from build123d import *


with BuildPart() as part:
    # Sketch1 → BaseBody (revolve)
    with BuildSketch(Plane.XY, mode=Mode.PRIVATE) as basebody_sk:
        with BuildLine():
            Line((0, 25.4), (0, 34.1249))
            ThreePointArc((0, 34.1249), (0.464967985, 35.247432015), (1.5875, 35.7124))
            Line((1.5875, 35.7124), (9.525, 35.7124))
            Line((9.525, 35.7124), (9.525, 30.35935))
            ThreePointArc((9.525, 30.35935), (8.263274015, 27.313274015), (11.30935, 28.575))
            Line((11.30935, 28.575), (71.2390625, 28.575))
            Line((71.2390625, 28.575), (73.025, 26.7890625))
            Line((73.025, 26.7890625), (73.025, 22.225))
            Line((73.025, 22.225), (3.175, 22.225))
            ThreePointArc((3.175, 22.225), (0.92993597, 23.15493597), (0, 25.4))
        make_face()
    revolve(basebody_sk.sketch.rotate(Axis((0, 0, 0), (1, 0, 0)), 90), axis=Axis((0, 0, 0), (1, 0, 0)))


solid = part.part
Input: part model. Units: mm. Frame: model coordinates. A direction names the side the tool comes from. Coordinates: 2 decimals unless noted, no trailing zeros. Loops run counter-clockwise (first coordinate to the right, second up) from the corner with the lowest first, then second, coordinate; pieces in that order, holes last.
Q1. Cut plane C-C (x = 21.5). Output: boundary loops of the cut face in (y, z) (3 decimals).
Q2. Draft query along Z for faces 1 (the face through (0, 2.37, 25.44)), 2 (the face through (37.6, -15, -16.4)), 3 (the face through (5.612, -10.727, 34.063)). Return one class per face: +Z half, -Z half, draft (parallel to the pull), parting line (faces both ways), or undercut.
Q3. Contact query for flat-ended pins moving along their axis: pin 1 (6 mm diameter, centred on x = 21, z = 5.5, fed in from -Y); pin 2 (5 mm diameter, centred on x = 50, z = -27, fed in from -Y); pin 3 (1.5 mm diameter, centred on x = 20.5, y = 21, fed in from -Z). Output: stop coordinate, or through.
Q4. Material intervals for line 1 (Y direction, x = 40, z = 0) (3 decimals); line 2 (Z direction, x = 9, y = -9.5); line 3 (X direction, y = 30.5, z = 15) (3 decimals), sorted ascending.
Q5. Set-up query: faces 4 (the face through (73.025, -16, -16)), 5 (the face through (9.525, 26, -16)). Return all of +Z, -Z, +X, -X, +Y, -Y with unobstructed straight access to the full face (end or side cutting, diameter ignored); none if empty.
Working result:
1. outline: circle Ø57.15 at (0, 0); hole circle Ø44.45 at (0, 0)
2. face 1: draft
2. face 2: undercut
2. face 3: parting line
3. pin 1: stops at y = -28.47
3. pin 2: stops at y = -14.71
3. pin 3: stops at z = -20.16
4. line 1: y = -28.575 to -22.225, 22.225 to 28.575
4. line 2: z = -34.43 to -28.75, -25.13 to -20.09, 20.09 to 25.13, 28.75 to 34.43
4. line 3: x = 0 to 9.525
5. face 4: +Z, -Z, +X, +Y, -Y
5. face 5: +X
